```python
from build123d import *

# Parameters (mm, degrees)
F0_W     = 87.369591
F0_H     = 53.756926
F1_DEPTH = 52.832
F2_R     = 20.235938
F4_D     = 2.54


with BuildPart() as f1:
    # F0 (on Top) → F1 (new body)
    with BuildSketch(Plane.XY):
        with Locations((0.62067, -1.921026)):
            Rectangle(F0_W, F0_H)
    extrude(amount=F1_DEPTH)

    # F2
    f2_edges = [f1.edges().sort_by_distance(p)[0] for p in [
        (0.620671, -28.799489, 52.832),
        (0.620671, 24.957437, 52.832),
        (44.305466, -1.921026, 52.832),
        (-43.064125, -1.921026, 52.832),
    ]]
    fillet(f2_edges, radius=F2_R)

    # F4 (through all)
    with Locations(Plane.XY.offset(52.832)):
        with Locations((-15.424626, -1.575627), (-6.023078, -1.575627), (4.138236, -1.575627), (16.751727, -1.575627)):
            Hole(F4_D / 2)


solid = f1.part
```
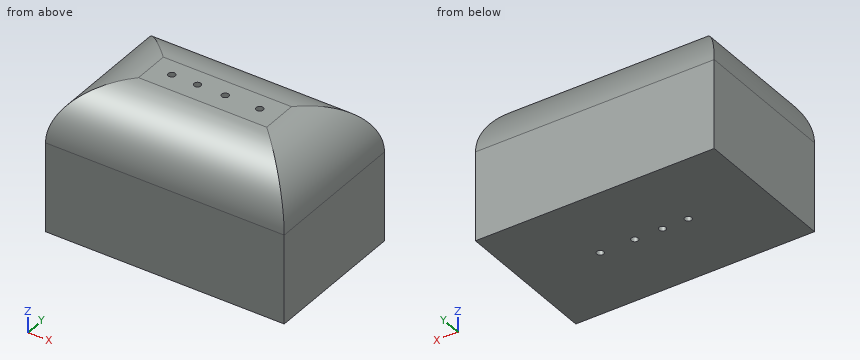
The listing builds one solid part. Answer for the finished solid, in the listing's coordinates (mm). Round coordinates to 2 decimals unless told otherwise and drop trailing zeros. Write each loop counter-clockwise with the first axis right and the second up, starting at its lowest first coordinate (ties: lowest second). Pieces come first, ordered by that corner, then holes. Notation, with made-up numbers: (63.5, -28.75) -> (107.5, -28.75) arc R17 ccw to (107.5, -12.75) -> close; hole circle Ø11 at (6, 80). An arc over 180 degrees is marked (long way). Use CSV: the item, a comma, the result in double quotes. Start each with the question number.
(1) Section C-C on y = -23.5 is taken. Give the vertices of the cut face in (x, z).
(2) Each of these flat-tipped pins is pushed along its axis until it touches: pin 1 (6 mm diameter, centred on x = -9, y = 12, fed in from +Z); pin 2 (4 mm diameter, centred on x = 31, y = -21, fed in from +Z); pin 3 (8 mm diameter, centred on x = 14, y = -18, fed in from +Z). Where does it stop, or does it pass through?
(3) Section A-A on z = 47 is taken. Give the vertices of the cut face in (x, y).
(4) Section B-B on x = -3 is taken. Give the vertices of the cut face in (y, z), then the cut area to 3 significant figures.
(5) Consider L1, parallel to Y at x = 16.5, z = 45; L2, parallel to Y at x = -8, z = 48.5; L3, parallel to Z at x = -21.5, y = -12.5. Determine where each line is inside the solid, lowest interval first. Write a range as from..to.
A:
1,outline,"(-43.06, 0) -> (44.31, 0) -> (44.31, 32.6) arc R20.24 ccw to (39.01, 46.25) -> (-37.76, 46.25) arc R20.24 ccw to (-43.06, 32.6) -> close"
2,pin 1,"stops at z = 52.37"
2,pin 2,"stops at z = 49.93"
2,pin 3,"stops at z = 52.09"
3,outline,"(-37.04, -22.78) -> (38.28, -22.78) -> (38.28, 18.93) -> (-37.04, 18.93) -> close; hole circle Ø2.54 at (-15.42, -1.58); hole circle Ø2.54 at (-6.02, -1.58); hole circle Ø2.54 at (4.14, -1.58); hole circle Ø2.54 at (16.75, -1.58)"
4,outline,"(-28.8, 0) -> (24.96, 0) -> (24.96, 32.6) arc R20.24 ccw to (4.72, 52.83) -> (-8.56, 52.83) arc R20.24 ccw to (-28.8, 32.6) -> close"
4,area,"2,660 mm²"
5,L1,"y = -24.55..-2.82, -0.33..20.71"
5,L2,"y = -21.08..17.23"
5,L3,"z = 0..52.45"
